Design review of the part built by this model. Coordinates are the model's own, in mm. Face numbers are marked on the shaded views. Coordinates: 2 decimals unless noted, no trailing zeros. Write each loop counter-clockwise with the first axis right and the second up, starting at its lowest first coordinate (ties: lowest second). Pieces come first, ordered by that corner, then holes.
Q1. Take a section at A-A (y = 1.5). Give the boundary of the cut face in (x, z), and give its area (3 significant figures).
Q2. Take a section at D-D (z = 1.75). Give the boundary of the cut face in (x, y).
Q3. Mouldability with a two-part tool opening along Y and no side actions: class the marked faces 1, 2 and 3 as pulls with the +Y half, pulls with the -Y half, needs draft (parallel to the pull), parting line crosses it, or undercut.
Q4. Take a section at B-B (x = -1.25). Give the boundary of the cut face in (y, z).
Q5. For probe 1 along Y at (x, z) = (-2.45, 0); probe 2 along Z at (x, y) = (-2.25, 1.5); probe 3 along X at (y, z) = (0.25, 0), list the stretches that pass through material, from the lowest coordinate up.
Q6. Insertion check: pin 1 (1 mm diameter, centred on x = 2, z = 2.5, fed in from +Y); pin 2 (0.8 mm diameter, centred on y = 2, z = 0, fed in from +X); pin 3 (1.5 mm diameter, centred on y = 1, z = 2.5, fed in from +X). Each pin has a flat end and moves straight along its axis. Give the tip position at first contact, or say it passes through.
Q7. Take a section at C-C (z = 0.75). Give the boundary of the cut face in (x, y).
```python
from build123d import *

# Parameters (mm, degrees)
SKETCH1_R           = 2.5
BOSS_EXTRUDE1_DEPTH = 0.5
SKETCH2_R           = 1.5
SKETCH2_R_2         = 1
BOSS_EXTRUDE2_DEPTH = 5


with BuildPart() as part:
    # Sketch1 → Boss-Extrude1 (new body)
    with BuildSketch(Plane(origin=(0, 0, 0), x_dir=(1, 0, 0), z_dir=(0, 1, 0))):
        with BuildLine():
            Line((0, -1), (0, 1))
            Line((0, 1), (1.5, 1))
            ThreePointArc((1.5, 1), (10.286184959, 0), (1.5, -1))
            Line((1.5, -1), (0, -1))
        make_face()
        with Locations((5.836184959, 0)):
            Circle(SKETCH1_R, mode=Mode.SUBTRACT)
    extrude(amount=BOSS_EXTRUDE1_DEPTH)

    # Sketch2 → Boss-Extrude2 (add)
    with BuildSketch(Plane(origin=(0, 0, 0), x_dir=(0, 0, -1), z_dir=(1, 0, 0))):
        with Locations((0, 1.5)):
            Circle(SKETCH2_R)
        with Locations((0, 1.5)):
            Circle(SKETCH2_R_2, mode=Mode.SUBTRACT)
    extrude(amount=-BOSS_EXTRUDE2_DEPTH)


solid = part.part
```
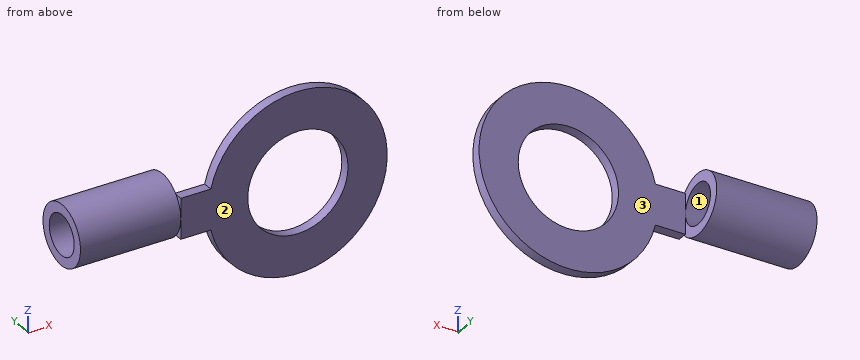
Response:
1. outline: (-5, -1.5) - (0, -1.5) - (0, -1) - (-5, -1) - close; (-5, 1) - (0, 1) - (0, 1.5) - (-5, 1.5) - close
1. area: 5.00 mm2
2. outline: (1.74, 0) - (4.05, 0) - (4.05, 0.5) - (1.74, 0.5) - close; (7.62, 0) - (9.93, 0) - (9.93, 0.5) - (7.62, 0.5) - close
3. face 1: undercut
3. face 2: pulls with the -Y half
3. face 3: pulls with the +Y half
4. outline: circle Ø3 at (1.5, 0); hole circle Ø2 at (1.5, 0)
5. probe 1: y = 0 to 0.5, 2.5 to 3
5. probe 2: z = -1.5 to -1, 1 to 1.5
5. probe 3: x = -5 to 3.34, 8.34 to 10.29
6. pin 1: stops at y = 0.5
6. pin 2: passes through
6. pin 3: stops at x = 9.84
7. outline: (-5, 0.2) - (0, 0.2) - (0, 0) - (3.45, 0) - (3.45, 0.5) - (0, 0.5) - (0, 0.84) - (-5, 0.84) - close; (-5, 2.16) - (0, 2.16) - (0, 2.8) - (-5, 2.8) - close; (8.22, 0) - (10.22, 0) - (10.22, 0.5) - (8.22, 0.5) - close
